Work out the finished part from the listing and answer in its coordinate system (mm). A direction names the side the tool comes from. Give positions to 0.01 mm unless a question says otherwise; leave off trailing zeros. Order: outer loops, then holes, each group sorted by start corner. A loop starts at its lowest first (then second) coordinate and runs counter-clockwise, first axis right, second up.
```python
from build123d import *

# Parameters (mm, degrees)
F1_DEPTH = 63.5
F0_W     = 25.4
F0_H     = 19.05
F2_DEPTH = 25.4
F3_DEPTH = 7.9375
F5_R     = 6.35


# Not quite as in the source:
# - a feature names something its author has since deleted; it is built from what else it names


with BuildPart() as f1:
    # F0 (on Front) → F1 (new body, symmetric)
    with BuildSketch(Plane.XZ):
        Polygon((-41.275, 9.525), (-41.275, -9.525), (41.275, -9.525), (41.275, 9.525), (22.225, 9.525), align=None)
    extrude(amount=F1_DEPTH, both=True)

    # F0 (on Front) → F2 (join, symmetric)
    with BuildSketch(Plane.XZ):
        with Locations((73.025, 52.3875)):
            Rectangle(F0_W, F0_H)
        with BuildLine():
            Line((22.225, 9.525), (41.275, 9.525))
            Line((41.275, 9.525), (41.275, 26.9875))
            ThreePointArc((41.275, 26.9875), (45.9246798487, 38.2128201513), (57.15, 42.8625))
            Line((57.15, 42.8625), (60.325, 42.8625))
            Line((60.325, 42.8625), (60.325, 61.9125))
            Line((60.325, 61.9125), (57.15, 61.9125))
            ThreePointArc((57.15, 61.9125), (32.4542956671, 51.6832043329), (22.225, 26.9875))
            Line((22.225, 26.9875), (22.225, 9.525))
        make_face()
    extrude(amount=F2_DEPTH, both=True)

    # F0 (on Front) → F3 (join, symmetric)
    with BuildSketch(Plane.XZ):
        with BuildLine():
            add(Edge.make_bspline(
                [(-41.275, 9.525), (-40.6160876155, 40.568407625), (17.4937602133, 61.9470998645), (57.15, 61.9125)],
                knots=[0, 0, 0, 0, 111.4985685166, 111.4985685166, 111.4985685166, 111.4985685166], degree=3))
            Line((-41.275, 9.525), (22.225, 9.525))
            Line((22.225, 9.525), (22.225, 26.9875))
            ThreePointArc((22.225, 26.9875), (32.4542956671, 51.6832043329), (57.15, 61.9125))
        make_face()
    extrude(amount=F3_DEPTH, both=True)

    # F0 (on Front) → F4 (revolve)
    with BuildSketch(Plane.XZ):
        Polygon((85.725, 66.675), (85.725, 61.9125), (85.725, 42.8625), (85.725, 38.1), (111.125, 38.1), (111.125, 66.675), align=None)
    revolve(axis=Axis((85.725, 0, 52.3875), (0, 0, 1)))

    # F5
    f5_edges = [f1.edges().sort_by_distance(p)[0] for p in [
        (41.275, -63.5, 0),
        (-41.275, -63.5, 0),
        (41.275, 63.5, 0),
        (-41.275, 63.5, 0),
    ]]
    fillet(f5_edges, radius=F5_R)


solid = f1.part
```
1. The part is cut by section D-D (y = 43). Write down the section's boundary in (x, z) (3 decimals), then the cut area to 3 significant figures.
Findings below:
outline: (-41.275, -9.525) - (41.275, -9.525) - (41.275, 9.525) - (-41.275, 9.525) - close
area: 1,570 mm2
2. The mould has two halves that part along X. Classify faces 1 (the face through (45.802, -0.356, 38.089)), 2 (the face through (39.464, -61.59, 0.133)), 3 (the face through (-1, -1, -9.525)), 4 (the face through (-39.464, 61.59, -0.133)): pulls with the +X half, pulls with the -X half, needs draft (parallel to the pull), parting line crosses it, or undercut.
Findings below:
face 1: undercut
face 2: pulls with the +X half
face 3: needs draft
face 4: pulls with the -X half
3. The part is cut by section A-A (z = -1.5). Write down the section's boundary in (x, y) (3 decimals), then the cut area to 3 significant figures.
Findings below:
outline: (-41.275, -57.15) arc R6.35 ccw to (-34.925, -63.5) - (34.925, -63.5) arc R6.35 ccw to (41.275, -57.15) - (41.275, 57.15) arc R6.35 ccw to (34.925, 63.5) - (-34.925, 63.5) arc R6.35 ccw to (-41.275, 57.15) - close
area: 10,400 mm2
4. Straight lines are drawn through the part: probe 1 along Z at (x, y) = (24.5, 25.5) (3 decimals); probe 2 along Y at (x, z) = (-1.5, 10.5); probe 3 along X at (y, z) = (37.5, -4.5) (3 decimals). For each, find the intervals that lie inside material, in ascending order.
Findings below:
probe 1: z = -9.525 to 9.525
probe 2: y = -7.94 to 7.94
probe 3: x = -41.275 to 41.275
5. The part is cut by section C-C (x = 80.5). Write down the section's boundary in (y, z) (1 decimal).
Findings below:
outline: (-25.4, 42.9) - (-24.9, 42.9) - (-24.9, 38.1) - (24.9, 38.1) - (24.9, 42.9) - (25.4, 42.9) - (25.4, 61.9) - (24.9, 61.9) - (24.9, 66.7) - (-24.9, 66.7) - (-24.9, 61.9) - (-25.4, 61.9) - close
6. Given P1, Ø16.5, axis at x = -15.5, y = 25, coming from the +Z side (3 decimals); P2, Ø5, axis at y = 10.5, z = 43.5, coming from the -X side; P3, Ø1, axis at y = -13, z = 36.5, coming from the -X side, each flat-ended and moving along its own axis, determine where each tip first touches the part or whether it passes through.
Findings below:
P1: stops at z = 9.525
P2: stops at x = 25.16
P3: stops at x = 23.41
7. Which of the six approach directions +Z, -Z, +X, -X, +Y, -Y give full straight-line access (tool end or side, diameter ignored) to faces 5 (the face through (60, -2, 61.912)), 6 (the face through (46, 25.4, 42)), 7 (the face through (32.727, 16.547, 51.953)), 8 (the face through (-2, -7.938, 30)), 9 (the face through (41.275, -1, 4))?
Findings below:
face 5: +Z, -X
face 6: +Z, +X, -X, +Y
face 7: +Z, -X, +Y
face 8: +Z, -X, -Y
face 9: -Z, +X, +Y, -Y
